Can you work these out from the model? Positions are in its coordinate system, mm. Round coordinates to 2 decimals unless told otherwise and drop trailing zeros. Loops run counter-clockwise (first coordinate to the right, second up) from the corner with the lowest first, then second, coordinate; pieces in that order, holes last. Notation, with made-up numbers: (-37.75, 32) - (-3.75, 32) arc R21 cw to (-3.75, 68) - close; hole circle Ø3 at (26, 33.25). An arc over 180 degrees is marked (long way). Answer as CSV lines item,"result".
```python
from build123d import *

# Parameters (mm, degrees)
EXTRUDE_1_DEPTH = 337
FILLET_1_R      = 25
FILLET_2_R      = 10


with BuildPart() as part:
    # 스케치1 → 보스-돌출1 (new body)
    with BuildSketch(Plane(origin=(0, 0, 0), x_dir=(1, 0, 0), z_dir=(0, 1, 0))):
        with BuildLine():
            Line((0, 0), (0, 800))
            Line((0, 800), (48, 800))
            ThreePointArc((48, 800), (118.710678119, 770.710678119), (148, 700))
            Line((148, 700), (148, 0))
            Line((148, 0), (0, 0))
        make_face()
    extrude(amount=EXTRUDE_1_DEPTH)

    # 필렛1
    fillet_1_edges = [part.edges().sort_by_distance(p)[0] for p in [
        (118.710678119, 337, -770.710678119),
        (24, 337, -800),
        (148, 337, -350),
    ]]
    fillet(fillet_1_edges, radius=FILLET_1_R)

    # 필렛2
    fillet_2_edges = [part.edges().sort_by_distance(p)[0] for p in [
        (148, 156, 0),
        (140.67766953, 329.67766953, 0),
        (61.5, 337, 0),
    ]]
    fillet(fillet_2_edges, radius=FILLET_2_R)


solid = part.part
```
Q1. If I drill on line 1 along Z through (x, y) = (53.5, 57); line 2 along X through (y, z) = (39, -705.5); line 3 along Z through (x, y) = (90.5, 86), over which ranges is the centre line in solid material (lowest first)? Write a range as [from, to].
Checks:
line 1,"[-799.85, 0]"
line 2,"[0, 147.85]"
line 3,"[-790.52, 0]"
Q2. Imagine slicing it at A-A (y = 255). Write out the boundary of the cut face in (x, z), then the cut area to 3 significant figures.
Checks:
outline,"(0, -800) - (48, -800) arc R100 ccw to (148, -700) - (148, -10) arc R10 ccw to (138, 0) - (0, 0) - close"
area,"116,000 mm²"
Q3. I'm going to push flat-ended pins straight in: pin 1 Ø5 at (x, z) = (72.5, -430) entering from -Y; pin 2 Ø3 at (x, z) = (126.5, -360) entering from +Y. Where does each tip first touch, or does it pass through?
Checks:
pin 1,"y = 0"
pin 2,"y = 336.92"
